Read the model definition and answer for the solid it produces. Units are mm, in the model's axes. Give positions to 0.01 mm unless a question says otherwise; leave off trailing zeros. Write each loop counter-clockwise with the first axis right and the second up, starting at its lowest first coordinate (ties: lowest second). Pieces come first, ordered by that corner, then holes. Notation, with made-up numbers: (-1, 80.25) - (29, 80.25) arc R25 cw to (29, 104.25) - close; hole circle Ø4 at (16, -11.75). An arc over 180 degrees is marked (long way). Answer as CSV lines item,"result".
```python
from build123d import *
from OCP.BRepFilletAPI import BRepFilletAPI_MakeChamfer

# Parameters (mm, degrees)
SKETCH1_W           = 72.39
SKETCH1_H           = 35.3568
BOSS_EXTRUDE1_DEPTH = 86.614
FILLET1_R           = 7.112
FILLET2_R           = 2.032
CUT_EXTRUDE1_DEPTH  = 17.0561
FILLET3_R           = 1.651
SKETCH3_W           = 1.8796
SKETCH3_H           = 4.572
BOSS_EXTRUDE2_DEPTH = 15.7861
SKETCH4_W           = 15.4432
SKETCH4_H           = 4.572
CUT_EXTRUDE2_DEPTH  = 3.175
CHAMFER1_SIZE       = 2.54
CHAMFER1_SIZE2      = 0.924484395
SKETCH5_R           = 7.62
BOSS_EXTRUDE3_DEPTH = 25.4
BOSS_EXTRUDE3_TAPER = 3.5
SKETCH7_R           = 3.2385
BOSS_EXTRUDE4_DEPTH = 32.766
SKETCH8_R           = 10.8966
BOSS_EXTRUDE5_DEPTH = 34.417
FILLET4_R           = 0.635
SKETCH9_R           = 3.2385
BOSS_EXTRUDE6_DEPTH = 34.417
SKETCH10_R          = 27.900404375
CUT_EXTRUDE3_DEPTH  = 83.82


with BuildPart() as part:
    # Sketch1 → Boss-Extrude1 (new, symmetric)
    with BuildSketch(Plane.XY):
        Rectangle(SKETCH1_W, SKETCH1_H)
    extrude(amount=BOSS_EXTRUDE1_DEPTH, both=True)

    # Fillet1
    fillet1_edges = [part.edges().sort_by_distance(p)[0] for p in [
        (36.195, 0, 86.614),
        (-36.195, 0, 86.614),
        (36.195, 0, -86.614),
        (-36.195, 0, -86.614),
    ]]
    fillet(fillet1_edges, radius=FILLET1_R)

    # Fillet2
    fillet2_edges = [part.edges().sort_by_distance(p)[0] for p in [
        (36.195, 17.6784, 0),
        (36.195, -17.6784, 0),
        (0, 17.6784, -86.614),
        (-36.195, 17.6784, 0),
        (0, 17.6784, 86.614),
        (-34.111943428, 17.6784, 84.530943428),
        (34.111943428, 17.6784, 84.530943428),
        (-34.111943428, 17.6784, -84.530943428),
        (34.111943428, 17.6784, -84.530943428),
        (0, -17.6784, -86.614),
        (0, -17.6784, 86.614),
        (-36.195, -17.6784, 0),
        (-34.111943428, -17.6784, 84.530943428),
        (34.111943428, -17.6784, 84.530943428),
        (-34.111943428, -17.6784, -84.530943428),
        (34.111943428, -17.6784, -84.530943428),
    ]]
    fillet(fillet2_edges, radius=FILLET2_R)

    # Sketch2 → Cut-Extrude1 (cut)
    with BuildSketch(Plane.XY.offset(86.614)):
        Polygon((7.47395, 9.0551), (-7.47395, 9.0551), (-11.938, 3.4544), (-11.938, -7.8359), (11.938, -7.8359), (11.938, 3.4544), align=None)
    extrude(amount=-CUT_EXTRUDE1_DEPTH, mode=Mode.SUBTRACT)

    # Fillet3
    fillet3_edges = [part.edges().sort_by_distance(p)[0] for p in [
        (11.938, -7.8359, 78.08595),
        (-11.938, -7.8359, 78.08595),
    ]]
    fillet(fillet3_edges, radius=FILLET3_R)

    # Sketch3 → Boss-Extrude2 (add)
    with BuildSketch(Plane.XY.offset(69.5579)):
        with Locations((-6.7818, -2.5019)):
            Rectangle(SKETCH3_W, SKETCH3_H)
        with Locations((0, 2.3876)):
            Rectangle(SKETCH3_W, SKETCH3_H)
        with Locations((6.7818, -2.5019)):
            Rectangle(SKETCH3_W, SKETCH3_H)
    extrude(amount=BOSS_EXTRUDE2_DEPTH)

    # Sketch4 → Cut-Extrude2 (cut)
    with BuildSketch(Plane.XY.offset(85.344)):
        with Locations((0, -2.5019)):
            Rectangle(SKETCH4_W, SKETCH4_H)
    extrude(amount=-CUT_EXTRUDE2_DEPTH, mode=Mode.SUBTRACT)

    # Chamfer1: one chamfer whose edges measure the first distance from different faces: ONE call of the kernel's chamfer builder (chamfer() names one face for all edges)
    chamfer1_edges_1 = [part.edges().sort_by_distance(p)[0] for p in [
        (0, 4.6736, 85.344),
    ]]
    chamfer1_side_1 = [part.faces().sort_by_distance(p)[0] for p in [
        (0, 4.6736, 77.45095),
    ]]
    chamfer1_edges_2 = [part.edges().sort_by_distance(p)[0] for p in [
        (0, 0.1016, 85.344),
    ]]
    chamfer1_side_2 = [part.faces().sort_by_distance(p)[0] for p in [
        (0, 0.1016, 77.45095),
    ]]
    chamfer1_edges_3 = [part.edges().sort_by_distance(p)[0] for p in [
        (-6.7818, -0.2159, 82.169),
    ]]
    chamfer1_side_3 = [part.faces().sort_by_distance(p)[0] for p in [
        (-6.7818, -0.2159, 75.86345),
    ]]
    chamfer1_edges_4 = [part.edges().sort_by_distance(p)[0] for p in [
        (6.7818, -0.2159, 82.169),
    ]]
    chamfer1_side_4 = [part.faces().sort_by_distance(p)[0] for p in [
        (6.7818, -0.2159, 75.86345),
    ]]
    chamfer1_edges_5 = [part.edges().sort_by_distance(p)[0] for p in [
        (-6.7818, -4.7879, 82.169),
    ]]
    chamfer1_side_5 = [part.faces().sort_by_distance(p)[0] for p in [
        (-6.7818, -4.7879, 75.86345),
    ]]
    chamfer1_edges_6 = [part.edges().sort_by_distance(p)[0] for p in [
        (6.7818, -4.7879, 82.169),
    ]]
    chamfer1_side_6 = [part.faces().sort_by_distance(p)[0] for p in [
        (6.7818, -4.7879, 75.86345),
    ]]
    chamfer1 = BRepFilletAPI_MakeChamfer(part.part.solid().wrapped)
    for e in chamfer1_edges_1:
        chamfer1.Add(CHAMFER1_SIZE, CHAMFER1_SIZE2, e.wrapped, chamfer1_side_1[0].wrapped)  # the first distance lies on this face
    for e in chamfer1_edges_2:
        chamfer1.Add(CHAMFER1_SIZE, CHAMFER1_SIZE2, e.wrapped, chamfer1_side_2[0].wrapped)  # the first distance lies on this face
    for e in chamfer1_edges_3:
        chamfer1.Add(CHAMFER1_SIZE, CHAMFER1_SIZE2, e.wrapped, chamfer1_side_3[0].wrapped)  # the first distance lies on this face
    for e in chamfer1_edges_4:
        chamfer1.Add(CHAMFER1_SIZE, CHAMFER1_SIZE2, e.wrapped, chamfer1_side_4[0].wrapped)  # the first distance lies on this face
    for e in chamfer1_edges_5:
        chamfer1.Add(CHAMFER1_SIZE, CHAMFER1_SIZE2, e.wrapped, chamfer1_side_5[0].wrapped)  # the first distance lies on this face
    for e in chamfer1_edges_6:
        chamfer1.Add(CHAMFER1_SIZE, CHAMFER1_SIZE2, e.wrapped, chamfer1_side_6[0].wrapped)  # the first distance lies on this face
    add(Compound.cast(chamfer1.Shape()), mode=Mode.REPLACE)

    # Sketch5 → Boss-Extrude3 (add)
    with BuildSketch(Plane(origin=(0, 0, -86.614), x_dir=(-1, 0, 0), z_dir=(0, 0, -1))):
        Circle(SKETCH5_R)
    extrude(amount=BOSS_EXTRUDE3_DEPTH, taper=BOSS_EXTRUDE3_TAPER)

    # Sketch7 → Boss-Extrude4 (add)
    with BuildSketch(Plane(origin=(0, 0, -112.014), x_dir=(-1, 0, 0), z_dir=(0, 0, -1))):
        Circle(SKETCH7_R)
    extrude(amount=BOSS_EXTRUDE4_DEPTH)

    # Sketch8 → Boss-Extrude5 (add)
    with BuildSketch(Plane(origin=(0, 0, -144.78), x_dir=(-1, 0, 0), z_dir=(0, 0, -1))):
        Circle(SKETCH8_R)
    extrude(amount=BOSS_EXTRUDE5_DEPTH)

    # Fillet4
    fillet4_edges = [part.edges().sort_by_distance(p)[0] for p in [
        (10.8966, 0, -144.78),
        (10.8966, 0, -179.197),
    ]]
    fillet(fillet4_edges, radius=FILLET4_R)

    # Sketch9 → Boss-Extrude6 (add)
    with BuildSketch(Plane(origin=(0, 0, -179.197), x_dir=(-1, 0, 0), z_dir=(0, 0, -1))):
        Circle(SKETCH9_R)
    extrude(amount=BOSS_EXTRUDE6_DEPTH)

    # Sketch10 → Cut-Extrude3 (cut)
    with BuildSketch(Plane(origin=(0, 0, -213.614), x_dir=(-1, 0, 0), z_dir=(0, 0, -1))):
        Circle(SKETCH10_R)
    extrude(amount=-CUT_EXTRUDE3_DEPTH, mode=Mode.SUBTRACT)


solid = part.part
```
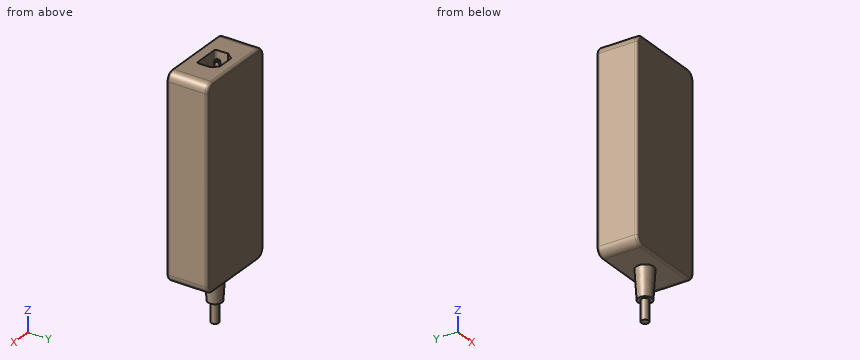
(1) A cutting plane is placed at B-B (y = -13). Write down the section's boundary in (x, z) (3 decimals).
Worked out:
outline,"(-36.195, -79.502) arc R7.112 ccw to (-29.083, -86.614) - (29.083, -86.614) arc R7.112 ccw to (36.195, -79.502) - (36.195, 79.502) arc R7.112 ccw to (29.083, 86.614) - (-29.083, 86.614) arc R7.112 ccw to (-36.195, 79.502) - close"
(2) Each of these flat-tipped pins is pushed along its axis until it touches: P1, Ø0.9, axis at x = -6.5, y = -3, coming from the +Z side; P2, Ø18.5, axis at x = -5, y = -2.5, coming from the +Z side; P3, Ø2, axis at x = 2.5, z = -94.5, coming from the +Y side; P4, Ø4, axis at x = 16, y = -3.5, coming from the -Z side. Where does it stop, or does it pass through?
Worked out:
P1,"stops at z = 82.17"
P2,"stops at z = 86.61"
P3,"stops at y = 6.99"
P4,"stops at z = -86.61"
(3) Find the intervals of material crossed by L1, parallel to Z at x = 5.5, y = 7.5; L2, parallel to Z at x = -28, y = -3.5; L3, parallel to X at y = 16, z = -59.5, in increasing order.
Worked out:
L1,"z = -86.61 to 69.56"
L2,"z = -86.61 to 86.61"
L3,"x = -36.16 to 36.16"
(4) A cutting plane is placed at A-A (x = 24.5). Write down the section's boundary in (y, z).
Worked out:
outline,"(-17.68, -84.58) arc R2.03 ccw to (-15.65, -86.61) - (15.65, -86.61) arc R2.03 ccw to (17.68, -84.58) - (17.68, 84.58) arc R2.03 ccw to (15.65, 86.61) - (-15.65, 86.61) arc R2.03 ccw to (-17.68, 84.58) - close"
